Source: CAD feature listing. Evaluate the final solid. Frame: model axes, mm. A direction names the side the tool comes from. Give positions to 0.01 mm unless a question says otherwise; leave off trailing zeros. Loops run counter-clockwise (first coordinate to the right, second up) from the corner with the lowest first, then second, coordinate; pieces in that order, holes last.
```python
from build123d import *

# Parameters (mm, degrees)
SKETCH1_R           = 4
SKETCH1_R_2         = 1.5
SKETCH1_W           = 5.2
SKETCH1_H           = 13.2
SKETCH1_W_2         = 13.2
SKETCH1_H_2         = 5.2
BOSS_EXTRUDE1_DEPTH = 5


with BuildPart() as part:
    # Sketch1 → Boss-Extrude1 (new body)
    with BuildSketch(Plane.XY):
        with BuildLine():
            Line((-6.232072687, 97.310592398), (-143.765004629, 97.310592398))
            ThreePointArc((-143.765004629, 97.310592398), (-147.300538535, 95.846126304), (-148.765004629, 92.310592398))
            Line((-148.765004629, 92.310592398), (-148.765004629, 16.510592398))
            ThreePointArc((-148.765004629, 16.510592398), (-147.300538535, 12.975058492), (-143.765004629, 11.510592398))
            Line((-143.765004629, 11.510592398), (-6.232072687, 11.510592398))
            ThreePointArc((-6.232072687, 11.510592398), (-2.696538781, 12.975058492), (-1.232072687, 16.510592398))
            Line((-1.232072687, 16.510592398), (-1.232072687, 92.310592398))
            ThreePointArc((-1.232072687, 92.310592398), (-2.696538781, 95.846126304), (-6.232072687, 97.310592398))
        make_face()
        with Locations((-74.998538658, 41.910592398)):
            Circle(SKETCH1_R, mode=Mode.SUBTRACT)
        with Locations((-83.998538658, 41.910592398)):
            Circle(SKETCH1_R_2, mode=Mode.SUBTRACT)
        with Locations((-65.998538658, 41.910592398)):
            Circle(SKETCH1_R_2, mode=Mode.SUBTRACT)
        with Locations((-8.835038658, 41.910592398)):
            Circle(SKETCH1_R_2, mode=Mode.SUBTRACT)
        with Locations(Location((-141.162038658, 41.910592398, 0), (0, 0, 180))):
            Circle(SKETCH1_R_2, mode=Mode.SUBTRACT)
        with Locations((-74.998538658, 64.310592398)):
            Circle(SKETCH1_R_2, mode=Mode.SUBTRACT)
        with Locations((-8.835038658, 26.110592398)):
            Rectangle(SKETCH1_W, SKETCH1_H, mode=Mode.SUBTRACT)
        with Locations((-8.835038658, 57.710592398)):
            Rectangle(SKETCH1_W, SKETCH1_H, mode=Mode.SUBTRACT)
        with Locations((-59.198538658, 64.310592398)):
            Rectangle(SKETCH1_W_2, SKETCH1_H_2, mode=Mode.SUBTRACT)
        with Locations((-90.798538658, 64.310592398)):
            Rectangle(SKETCH1_W_2, SKETCH1_H_2, mode=Mode.SUBTRACT)
        with Locations((-141.162038658, 57.710592398)):
            Rectangle(SKETCH1_W, SKETCH1_H, mode=Mode.SUBTRACT)
        with Locations((-141.162038658, 26.110592398)):
            Rectangle(SKETCH1_W, SKETCH1_H, mode=Mode.SUBTRACT)
    extrude(amount=BOSS_EXTRUDE1_DEPTH)


solid = part.part
```
(1) Section C-C, the plane z = 3.65. Count the separate pieces of the cut face and the enclosed holes in it, then the cut area to 3 significant figures.
A:
separate pieces: 1
enclosed holes: 12
area: 12,100 mm2
(2) Mould query, pull axis X, two halves, no side actions, for faces 1 (the flat face through (-76, 11.511, 2)), 2 (the flat face through (-138.562, 26, 2)), 3 (the cylindrical face through (-147.339, 13.014, 2.465)). Classes: pulls with the +X half, pulls with the -X half, needs draft (parallel to the pull), parting line crosses it, or undercut.
A:
face 1: needs draft
face 2: undercut
face 3: pulls with the -X half
(3) Ray query, line 1 along X through (y, z) = (26.5, 2.1) (3 decimals); line 2 along Y through (x, z) = (-89, 0.8); line 3 along Y through (x, z) = (-140, 1.75). Return the intervals inside material, ascending.
A:
line 1: x = -148.765 to -143.762, -138.562 to -11.435, -6.235 to -1.232
line 2: y = 11.51 to 61.71, 66.91 to 97.31
line 3: y = 11.51 to 19.51, 32.71 to 40.96, 42.86 to 51.11, 64.31 to 97.31
(4) Reachability of faces 4 (the flat face through (-11.435, 58, 2)), 5 (the flat face through (-74, 97.311, 2)) from +Z, -Z, +X, -X, +Y, -Y: full face, straight path, thin tool, end or side. Return the list, or none.
A:
face 4: +Z, -Z
face 5: +Z, -Z, +X, -X, +Y
(5) Section A-A, the plane x = -55. Return the cut outline in (y, z).
A:
outline: (11.51, 0) - (61.71, 0) - (61.71, 5) - (11.51, 5) - close; (66.91, 0) - (97.31, 0) - (97.31, 5) - (66.91, 5) - close
(6) Section B-B, the plane y = 22. Return the cut outline in (x, z) (3 decimals), then the cut area to 3 significant figures.
A:
outline: (-148.765, 0) - (-143.762, 0) - (-143.762, 5) - (-148.765, 5) - close; (-138.562, 0) - (-11.435, 0) - (-11.435, 5) - (-138.562, 5) - close; (-6.235, 0) - (-1.232, 0) - (-1.232, 5) - (-6.235, 5) - close
area: 686 mm2
